Could you check a few things on this model? Use its own coordinates, in mm. Face numbers are marked on the shaded views. A direction names the side the tool comes from. Give positions to 0.01 mm unless a question says otherwise; leave off trailing zeros. Order: outer loops, then holes, each group sorted by start corner. A loop starts at its lowest first (then second) coordinate and runs counter-clockwise, first axis right, second up. Notation, with made-up numbers: (67.25, 13) - (118.25, 13) arc R23 cw to (118.25, 50) - close; hole circle Ø5 at (64, -31). An arc over 180 degrees is marked (long way). Put each result on its own line as item: value.
from build123d import *

# Parameters (mm, degrees)
SKETCH2_W  = 15.85
SKETCH2_H  = 2.5
SKETCH5_R  = 22.25
STUB_DEPTH = 10.2
FILLET1_R  = 0.762
FILLET2_R  = 0.254


with BuildPart() as part:
    # Sketch1 → Flange (revolve)
    with BuildSketch(Plane(origin=(0, 0, 0), x_dir=(0, 0, -1), z_dir=(1, 0, 0)), mode=Mode.PRIVATE) as flange_sk:
        Polygon((-27.5, 0), (-27.5, 3.175), (-20.315802195, 5.1), (0, 5.1), (0, 2.5), (-20.625, 2.5), (-20.625, 0), align=None)
    revolve(flange_sk.sketch.rotate(Axis((0, 0, 0), (0, 1, 0)), 180), axis=Axis((0, 0, 0), (0, 1, 0)))

    # Sketch2 → Blank Insert (revolve)
    with BuildSketch(Plane(origin=(0, 0, 0), x_dir=(0, 0, -1), z_dir=(1, 0, 0))):
        with Locations((-7.925, 1.25)):
            Rectangle(SKETCH2_W, SKETCH2_H)
    revolve(axis=Axis((0, 0, 0), (0, -1, 0)))

    # Sketch5 → Stub (add)
    with BuildSketch(Plane.XZ.offset(-2.5)):
        with Locations(Location((0, 0, 0), (0, 0, 270))):
            Circle(SKETCH5_R)
    extrude(amount=-STUB_DEPTH)

    # Fillet1
    fillet1_edges = [part.edges().sort_by_distance(p)[0] for p in [
        (0, 3.175, 27.5),
    ]]
    fillet(fillet1_edges, radius=FILLET1_R)

    # Fillet2
    fillet2_edges = [part.edges().sort_by_distance(p)[0] for p in [
        (0, 0, 27.5),
    ]]
    fillet(fillet2_edges, radius=FILLET2_R)


solid = part.part
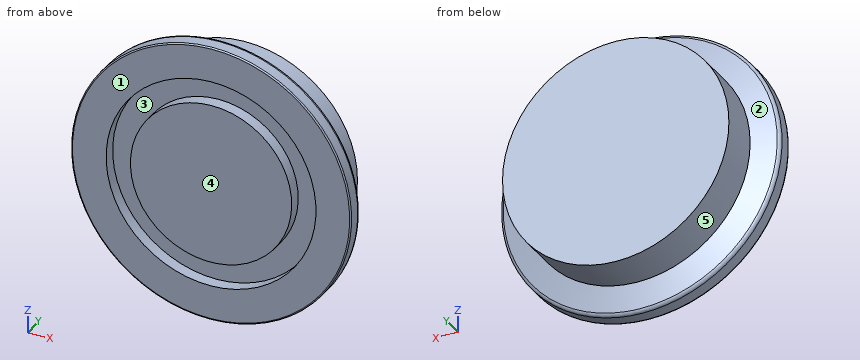
1) If I drill on line 1 (Z direction, x = 3, y = 0.5); line 2 (Y direction, x = -17, z = -5.5); line 3 (X direction, y = 1.25, z = -8.5), over which ranges is the centre line in solid material (lowest first)? Write a range as [from, to].
Filled in:
line 1: z = [-27.34, -20.41], [-15.56, 15.56], [20.41, 27.34]
line 2: y = [2.5, 12.7]
line 3: x = [-26.15, -18.79], [-13.38, 13.38], [18.79, 26.15]
2) We'd pull the mould along Z, two halves only. Please class the marked faces 1, 2 and 3: pulls with the +Z half, pulls with the -Z half, needs draft (parallel to the pull), parting line crosses it, or undercut.
Filled in:
face 1: needs draft
face 2: parting line crosses it
face 3: undercut
3) Suppose I cut it at A-A, the plane y = 8.75. List the corners of the cut face in (x, z) for me.
Filled in:
outline: circle Ø44.5 at (0, 0)
4) I'm going to push flat-ended pins straight in: pin 1 (1.5 mm diameter, centred on x = 4.5, y = 8, fed in from +Z); pin 2 (6 mm diameter, centred on y = 11.5, z = -18.5, fed in from -X); pin 3 (3 mm diameter, centred on y = 7, z = 11, fed in from +X). Where does each tip first touch, or does it pass through?
Filled in:
pin 1: stops at z = 21.93
pin 2: stops at x = -15.96
pin 3: stops at x = 20.12
5) Which directions (+Z, -Z, +X, -X, +Y, -Y) give clear straight access to the entire face, cutting with the end or side of a thin tool? Please do the marked faces 4 and 5.
Filled in:
face 4: +Z, -Z, +X, -X, -Y
face 5: +Y
